from build123d import *

# Parameters (mm, degrees)
SKETCH2_W          = 2.85
SKETCH2_H          = 2.85
CUT_EXTRUDE1_DEPTH = 2.5


with BuildPart() as part:
    # Sketch1 → Revolve1 (revolve)
    with BuildSketch(Plane.XY, mode=Mode.PRIVATE) as revolve1_sk:
        with BuildLine():
            Line((0, 0), (33, 0))
            Line((33, 0), (33, 2))
            Line((33, 2), (3, 2))
            Line((3, 2), (3, 2.875))
            ThreePointArc((3, 2.875), (2.707106781, 3.582106781), (2, 3.875))
            ThreePointArc((2, 3.875), (0.585786438, 3.289213562), (0, 1.875))
            Line((0, 1.875), (0, 0))
        make_face()
    revolve(revolve1_sk.sketch.rotate(Axis((0, 0, 0), (-1, 0, 0)), 90), axis=Axis((0, 0, 0), (-1, 0, 0)))

    # Sketch2 → Cut-Extrude1 (cut)
    with BuildSketch(Plane.ZY):
        Rectangle(SKETCH2_W, SKETCH2_H)
    extrude(amount=-CUT_EXTRUDE1_DEPTH, mode=Mode.SUBTRACT)


solid = part.part
Input: part model. Units: mm. Frame: model coordinates. A direction names the side the tool comes from. Round coordinates to 2 decimals unless told otherwise and drop trailing zeros. Loops run counter-clockwise (first coordinate to the right, second up) from the corner with the lowest first, then second, coordinate; pieces in that order, holes last. Notation, with made-up numbers: (3, 82) -> (17, 82) arc R24 ccw to (17, 109) -> close; hole circle Ø8 at (-13, 67.25). An arc over 180 degrees is marked (long way). Answer as a JSON object with one key per item and string values. Group by question number.
1) Reachability of faces 5 (the flat face through (2.5, 0, 0)), 6 (the flat face through (33, 0, 0)) from +Z, -Z, +X, -X, +Y, -Y: full face, straight path, thin tool, end or side. Return the list, or none.
2) Pin query (flat end, axial travel): pin 1 (2.5 mm diameter, centred on y = 0, z = 0, fed in from -X); pin 2 (1.5 mm diameter, centred on y = -3, z = -2, fed in from +X); pin 3 (0.8 mm diameter, centred on x = 2, y = 0.5, fed in from -Z); pin 4 (2 mm diameter, centred on x = 1, z = 0.5, fed in from +Y). Return the tip coordinate at first contact, or that it passes through.
3) Ray query, L1, parallel to X at y = 0, z = 0.5; L2, parallel to Y at x = 2, z = 0.5 (3 decimals); L3, parallel to Z at x = 12.5, y = 0.5. Return the intervals inside material, ascending.
4) Draft query along Z for faces 1 (the cylindrical face through (18, 2, 0)), 2 (the flat face through (1, 0, 1.425)), 3 (the flat face through (1, -1.425, 0)), 4 (the flat face through (3, 1, -2)). Return one class per face: +Z half, -Z half, draft (parallel to the pull), parting line (faces both ways), or undercut.
5) Section query A-A on x = 5.5. Output: boundary loops of the cut face in (y, z), plus the area to 3 significant figures.
Reply:
{
 "1": {"face 5": "-X", "face 6": "+Z, -Z, +X, +Y, -Y"},
 "2": {"pin 1": "stops at x = 2.5", "pin 2": "stops at x = 3", "pin 3": "stops at z = -3.87", "pin 4": "stops at y = 3.87"},
 "3": {"L1": "x = 2.5 to 33", "L2": "y = -3.843 to -1.425, 1.425 to 3.843", "L3": "z = -1.94 to 1.94"},
 "4": {"face 1": "parting line", "face 2": "undercut", "face 3": "undercut", "face 4": "draft"},
 "5": {"outline": "circle Ø4 at (0, 0)", "area": "12.6 mm2"}
}
